```python
from build123d import *

# Parameters (mm, degrees)
F1_DEPTH = 25.4
F2_DEPTH = 101.6
F3_R     = 12.7
F4_DEPTH = 25.4
F5_R     = 12.7
F6_DEPTH = 25.4


with BuildPart() as f1:
    # F0 (on Front) → F1 (new body)
    with BuildSketch(Plane.XZ):
        Polygon((64.253767, 80.411777), (-11.946233, 80.411777), (-11.946233, 29.611777), (-37.346233, 29.611777), (-37.346233, -21.188223), (64.253767, -21.188223), align=None)
    extrude(amount=F1_DEPTH)

    # F0 (on Front) → F2 (join)
    with BuildSketch(Plane.XZ):
        Polygon((64.253767, -97.725551), (64.253767, -21.188223), (-37.346233, -21.188223), (-37.346233, -46.588223), (38.856007, -46.588223), (38.856007, -97.388223), align=None)
    extrude(amount=F2_DEPTH)

    # F3 (on face) → F4 (cut)
    with BuildSketch(Plane.XZ.offset(25.4)):
        with Locations((26.153767, 42.311777)):
            Circle(F3_R)
    extrude(amount=-F4_DEPTH, mode=Mode.SUBTRACT)

    # F5 (on face) → F6 (cut)
    with BuildSketch(Plane(origin=(0, 0, -46.588223), x_dir=(1, 0, 0), z_dir=(0, 0, -1))):
        with Locations((0, 63.5)):
            Circle(F5_R)
    extrude(amount=-F6_DEPTH, mode=Mode.SUBTRACT)


solid = f1.part
```
The model under review builds one solid part; all positions refer to its coordinate system, in mm. A direction names the side the tool comes from. Give positions to 0.01 mm unless a question says otherwise; leave off trailing zeros. Write each loop counter-clockwise with the first axis right and the second up, starting at its lowest first coordinate (ties: lowest second). Pieces come first, ordered by that corner, then holes. Notation, with made-up numbers: (36.5, -4.5) - (55.5, -4.5) arc R18 cw to (55.5, 19.5) - close; hole circle Ø3 at (60.25, 51). An arc over 180 degrees is marked (long way). Answer in a Markdown table with one row per item. Add a question column.
1. We need section C-C on z = 46. Write out the cut boundary in (x, y), then the cut area to 3 significant figures.
2. We need section D-D on y = -39. Write out the cut boundary in (x, z).
3. Draft analysis for pull direction Z (two halves, no side actions). For faces 1 (the flat face through (0, -50, -46.588)), 2 (the cylindrical face through (38.267, -12.878, 46.127)), 3 (the flat face through (14, -63, -21.188)), 4 (the flat face through (-11.946, -13, 55)), state which applies: +Z half, -Z half, draft (parallel to the pull), parting line (faces both ways), or undercut.
4. Insertion check: P1, Ø7.5, axis at y = -9, z = 62.5, coming from the -X side; P2, Ø10, axis at y = -13, z = -76, coming from the -X side; P3, Ø8, axis at x = 5, z = -4.5, coming from the -Y side. Each pin has a flat end and moves straight along its axis. Give the tip position at first contact, or say it passes through.
5. We need section A-A on x = 0. Write out the cut boundary in (y, z), then the cut area to 3 significant figures.
6. Tool access review of faces 5 (the flat face through (13, -25.4, 30)), 6 (the flat face through (-24, -13, 29.612)), 7 (the flat face through (38.856, -50, -72)): name each direction out of +Z, -Z, +X, -X, +Y, -Y from which nothing blocks a thin tool from reaching the whole face with its end or side.
7. We need section B-B on y = -63.5. Write out the cut boundary in (x, z), then the cut area to 3 significant figures.
8. Wall thickness on line 1 along Y through (x, z) = (0, -26.25); line 2 along Y through (x, z) = (-32.5, 22); line 3 along Z through (x, y) = (-26.5, -62.5): over which ranges is each line inside the solid? List them lowest first. Write a range as [from, to].
Ans:
| question | item | result |
|---|---|---|
| 1 | outline | (-11.95, -25.4) - (14, -25.4) - (14, 0) - (-11.95, 0) - close; (38.31, -25.4) - (64.25, -25.4) - (64.25, 0) - (38.31, 0) - close |
| 1 | area | 1,320 mm^2 |
| 2 | outline | (-37.35, -46.59) - (38.86, -46.59) - (38.86, -97.39) - (64.25, -97.73) - (64.25, -21.19) - (-37.35, -21.19) - close |
| 3 | face 1 | -Z half |
| 3 | face 2 | undercut |
| 3 | face 3 | +Z half |
| 3 | face 4 | draft |
| 4 | P1 | stops at x = -11.95 |
| 4 | P2 | stops at x = 38.86 |
| 4 | P3 | stops at y = -25.4 |
| 5 | outline | (-101.6, -46.59) - (-76.2, -46.59) - (-76.2, -21.19) - (-101.6, -21.19) - close; (-50.8, -46.59) - (0, -46.59) - (0, 80.41) - (-25.4, 80.41) - (-25.4, -21.19) - (-50.8, -21.19) - close |
| 5 | area | 4,520 mm^2 |
| 6 | face 5 | +Z, +X, -X, -Y |
| 6 | face 6 | +Z, -X, +Y, -Y |
| 6 | face 7 | -Z, -X, +Y, -Y |
| 7 | outline | (-37.35, -46.59) - (-12.7, -46.59) - (-12.7, -21.19) - (-37.35, -21.19) - close; (12.7, -46.59) - (38.86, -46.59) - (38.86, -97.39) - (64.25, -97.73) - (64.25, -21.19) - (12.7, -21.19) - close |
| 7 | area | 3,230 mm^2 |
| 8 | line 1 | y = [-101.6, -76.2], [-50.8, 0] |
| 8 | line 2 | y = [-25.4, 0] |
| 8 | line 3 | z = [-46.59, -21.19] |
